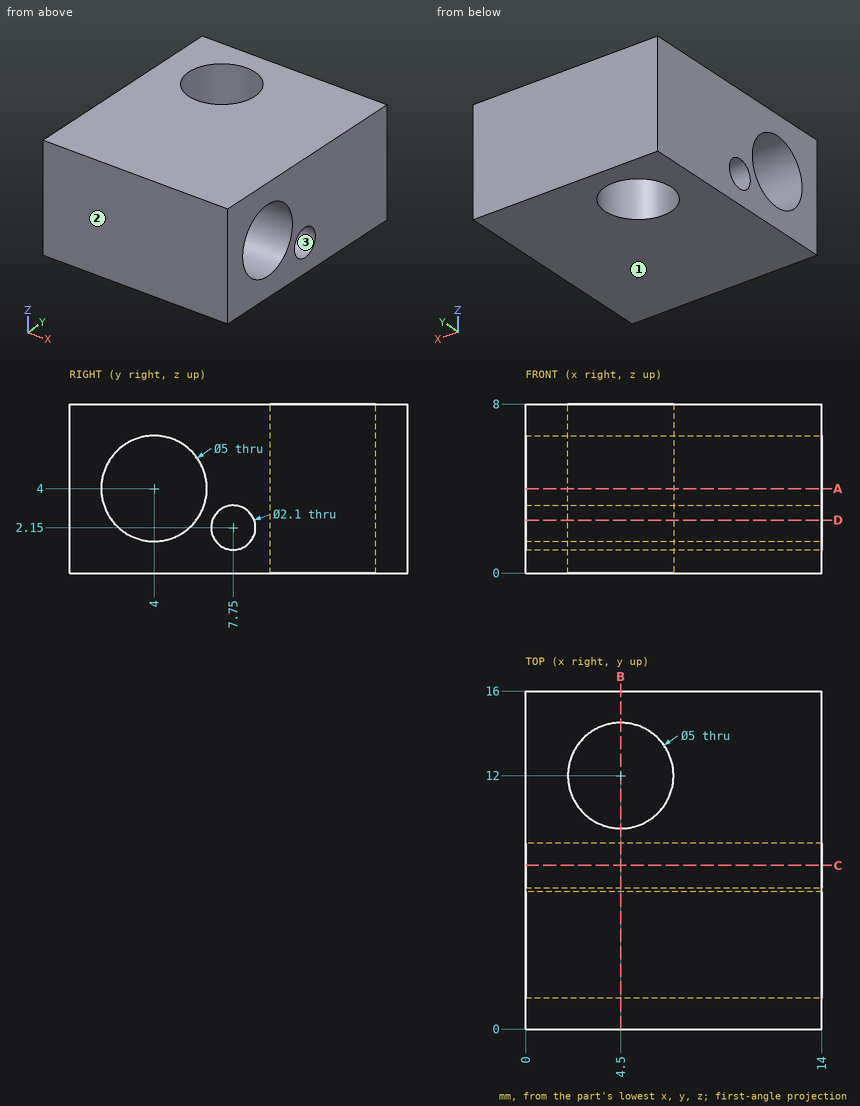
The figure shows three views and two pictorial views of one solid part (mm, origin at its lowest corner). Answer the questions. Round coordinates to 2 decimals unless told otherwise and drop trailing zeros. Write each loop counter-clockwise with the first axis right and the second up, starting at its lowest first coordinate (ties: lowest second). Pieces come first, ordered by that corner, then holes. Notation, with made-up numbers: (61.25, 74) - (95.25, 74) arc R22 ccw to (95.25, 94) - close; hole circle Ø5 at (75.25, -24.75). An arc over 180 degrees is marked (long way). Answer in a Markdown table with one row per item. Add a question column.
1. A cutting plane is placed at A-A, the plane z = 4. Determine the outline of the cut face in (x, y).
2. A cutting plane is placed at C-C, the plane y = 7.75. Determine the outline of the cut face in (x, z).
3. A cutting plane is placed at D-D, the plane z = 2.5. Determine the outline of the cut face in (x, y).
4. A cutting plane is placed at B-B, the plane x = 4.5. Determine the outline of the cut face in (y, z), and give its area (3 significant figures).
5. Find the intervals of material crossed by line 1 along Y through (x, z) = (5.25, 5); line 2 along Z through (x, y) = (3, 4); line 3 along Y through (x, z) = (1, 3), in increasing order. Write a range as from..to.
6. The mould has two halves that part along Z. Classify the marked faces 1, 2 and 3: +Z half, -Z half, draft (parallel to the pull), parting line (faces both ways), or undercut.
Worked out:
| question | item | result |
|---|---|---|
| 1 | outline | (0, 0) - (14, 0) - (14, 1.5) - (0, 1.5) - close; (0, 6.5) - (14, 6.5) - (14, 16) - (0, 16) - close; hole circle Ø5 at (4.5, 12) |
| 2 | outline | (0, 0) - (14, 0) - (14, 1.1) - (0, 1.1) - close; (0, 3.2) - (14, 3.2) - (14, 8) - (0, 8) - close |
| 3 | outline | (0, 0) - (14, 0) - (14, 2) - (0, 2) - close; (0, 6) - (14, 6) - (14, 6.76) - (0, 6.76) - close; (0, 8.74) - (14, 8.74) - (14, 16) - (0, 16) - close; hole circle Ø5 at (4.5, 12) |
| 4 | outline | (0, 0) - (9.5, 0) - (9.5, 8) - (0, 8) - close; (14.5, 0) - (16, 0) - (16, 8) - (14.5, 8) - close; hole circle Ø5 at (4, 4); hole circle Ø2.1 at (7.75, 2.15) |
| 4 | area | 64.9 mm^2 |
| 5 | line 1 | 0..1.71, 6.29..9.62, 14.38..16 |
| 5 | line 2 | 0..1.5, 6.5..8 |
| 5 | line 3 | 0..1.71, 6.29..7.13, 8.37..16 |
| 6 | face 1 | -Z half |
| 6 | face 2 | draft |
| 6 | face 3 | undercut |
